from build123d import *

# Parameters (mm, degrees)
SKETCH3_R           = 35.625
SKETCH3_R_2         = 25.625
BOSS_EXTRUDE1_DEPTH = 5
CUT_EXTRUDE1_REACH  = 52.629
SKETCH4_R           = 1.5
CIRPATTERN1_COUNT   = 12
CHAMFER1_SIZE       = 0.5


with BuildPart() as part:
    # Sketch3 → Boss-Extrude1 (new body)
    with BuildSketch(Plane(origin=(0, 0, 0), x_dir=(1, 0, 0), z_dir=(0, 1, 0))):
        with Locations(Location((0, 0, 0), (0, 0, 270))):
            Circle(SKETCH3_R)
        with Locations(Location((0, 0, 0), (0, 0, 270))):
            Circle(SKETCH3_R_2, mode=Mode.SUBTRACT)
    extrude(amount=BOSS_EXTRUDE1_DEPTH)

    # Sketch4 → Cut-Extrude1 (cut, up to next)
    with BuildSketch(Plane(origin=(0, 5, 0), x_dir=(1, 0, 0), z_dir=(0, 1, 0)), mode=Mode.PRIVATE) as cut_extrude1_sk1:
        with Locations(Location((0, 30.625, 0), (0, 0, 270))):
            Circle(SKETCH4_R)
    cut_extrude1_tool1 = extrude(cut_extrude1_sk1.sketch, amount=-CUT_EXTRUDE1_REACH, mode=Mode.PRIVATE) & part.part
    cut_extrude1 = cut_extrude1_tool1.solids().sort_by_distance((0, 5, -30.625))[0]
    add(cut_extrude1, mode=Mode.SUBTRACT)

    # CirPattern1: Cut-Extrude1 ×12 about axis
    cirpattern1_axis = Axis((0, 0, 0), (0, 1, 0))
    for i in range(1, CIRPATTERN1_COUNT):
        add(cut_extrude1.rotate(cirpattern1_axis, i * 360 / CIRPATTERN1_COUNT), mode=Mode.SUBTRACT)

    # Chamfer1
    chamfer1_edges = [part.edges().sort_by_distance(p)[0] for p in [
        (0, 0, -35.625),
        (0, 5, -35.625),
        (0, 0, -25.625),
        (0, 5, -25.625),
    ]]
    chamfer(chamfer1_edges, length=CHAMFER1_SIZE)


solid = part.part
Verification items for the finished model (mm, model axes). Coordinates: 2 decimals unless noted, no trailing zeros. Write each loop counter-clockwise with the first axis right and the second up, starting at its lowest first coordinate (ties: lowest second). Pieces come first, ordered by that corner, then holes. Notation, with made-up numbers: (19, 6) -> (65, 6) arc R20 ccw to (65, 32) -> close; hole circle Ø5 at (-21, 19). An arc over 180 degrees is marked (long way). One line per item, written item: value. Start each with the question number.
Q1. Mould release check, pull along Z, two halves, no side actions. Record for faces 1 (the cylindrical face through (-25.508, 2.535, 14.207)), 2 (the flat face through (26.2, 5, 2.4)), 3 (the cylindrical face through (-21.68, 2.47, -28.27)), 4 (the cylindrical face through (-25.058, 2.535, -14.987)): pulls with the +Z half, pulls with the -Z half, needs draft (parallel to the pull), parting line crosses it, or undercut.
Q2. Cross-section at A-A on z = 0. Enter the section's corners in (x, y) (3 decimals), and give its area (3 significant figures).
Q3. Go/stop test with flat-tipped pins: P1, Ø1, axis at y = 1, z = -12, coming from the -X side; P2, Ø1.5, axis at y = 2, z = 23.5, coming from the +X side; P3, Ø3, axis at x = 21.5, y = 3.5, coming from the +Z side. Record where each tip stops, or that it passes through.
Q4. Cross-section at B-B on x = 0. Enter the section's corners in (y, z) (3 decimals), and give its area (3 significant figures).
Q5. Thickness scan on L1, parallel to Z at x = -1, y = 1.75; L2, parallel to X at y = 1.45, z = 14; L3, parallel to X at y = 0.7, z = -26. Record the ranges inside material, lowest first. Write a range as from..to.
Q6. Cross-section at C-C on y = 2.7. State how many separate pieces and enclosed holes the cut face has, and give its area (3 significant figures).
Checked values:
1. face 1: undercut
1. face 2: needs draft
1. face 3: parting line crosses it
1. face 4: undercut
2. outline: (-35.625, 0.5) -> (-35.125, 0) -> (-32.125, 0) -> (-32.125, 5) -> (-35.125, 5) -> (-35.625, 4.5) -> close; (-29.125, 0) -> (-26.125, 0) -> (-25.625, 0.5) -> (-25.625, 4.5) -> (-26.125, 5) -> (-29.125, 5) -> close; (25.625, 0.5) -> (26.125, 0) -> (29.125, 0) -> (29.125, 5) -> (26.125, 5) -> (25.625, 4.5) -> close; (32.125, 0) -> (35.125, 0) -> (35.625, 0.5) -> (35.625, 4.5) -> (35.125, 5) -> (32.125, 5) -> close
2. area: 69.0 mm²
3. P1: stops at x = -33.72
3. P2: stops at x = 27.41
3. P3: stops at z = 29.48
4. outline: (0, -35.125) -> (0.5, -35.625) -> (4.5, -35.625) -> (5, -35.125) -> (5, -32.125) -> (0, -32.125) -> close; (0, -29.125) -> (5, -29.125) -> (5, -26.125) -> (4.5, -25.625) -> (0.5, -25.625) -> (0, -26.125) -> close; (0, 26.125) -> (0.5, 25.625) -> (4.5, 25.625) -> (5, 26.125) -> (5, 29.125) -> (0, 29.125) -> close; (0, 32.125) -> (5, 32.125) -> (5, 35.125) -> (4.5, 35.625) -> (0.5, 35.625) -> (0, 35.125) -> close
4. area: 69.0 mm²
5. L1: z = -35.61..-31.74, -29.51..-25.61, 25.61..29.51, 31.74..35.61
5. L2: x = -32.76..-27.25, -25.8..-21.46, 21.46..25.8, 27.25..32.76
5. L3: x = -24.35..-16.72, -13.91..13.91, 16.72..24.35
6. separate pieces: 1
6. enclosed holes: 13
6. area: 1,840 mm²
